Source: three-view drawing plus pictorial views. Frame: mm from the lowest corner of the part. Coordinates: 2 decimals unless noted, no trailing zeros. Order: outer loops, then holes, each group sorted by start corner. A loop starts at its lowest first (then second) coordinate and runs counter-clockwise, first axis right, second up. Notation, with made-up numbers: (81.5, -15) - (117.5, -15) arc R12 cw to (117.5, -1) - close; hole circle Ø4 at (-38, 64). An arc over 180 degrees is marked (long way). Use a Markdown table: item, result. Add a question column.
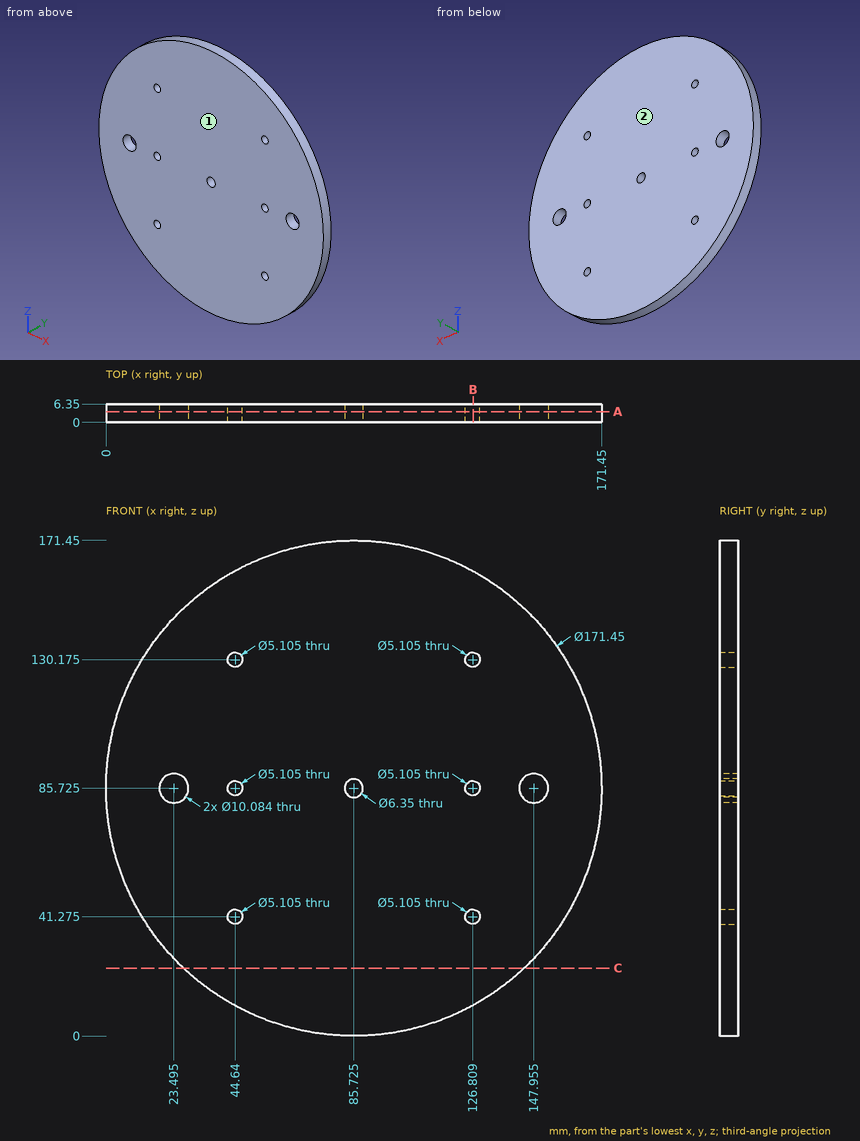
1) Section A-A (y = 3.75). Give the number of separate pieces and of enclosed holes in the cut face, then the cut area to 3 significant figures.
2) Section C-C (z = 23.5). Return loops of the section in (x, y), then the cut area to 3 significant figures.
3) Ray query, line 1 along X through (y, z) = (3, 43) (1 decimal); line 2 along X through (y, z) = (5, 130.5); line 3 along Z through (x, y) = (25, 5.75) (1 decimal). Return the intervals inside material, ascending.
4) Pin query (flat end, axial travel): pin 1 (1 mm diameter, centred on y = 4.5, z = 94.5, fed in from -X); pin 2 (3 mm diameter, centred on x = 107, y = 5.5, fed in from -Z); pin 3 (2 mm diameter, centred on x = 33.5, y = 2.5, fed in from +Z). Return the tip coordinate at first contact, or that it passes through.
5) Draft query along Y for the marked faces 1 and 2. Return one class per face: pulls with the +Y half, pulls with the -Y half, needs draft (parallel to the pull), parting line crosses it, or undercut.
6) Section B-B (x = 127). Return loops of the section in (y, z).
Values follow:
| question | item | result |
|---|---|---|
| 1 | separate pieces | 1 |
| 1 | enclosed holes | 9 |
| 1 | area | 22,800 mm² |
| 2 | outline | (26.76, 0) - (144.69, 0) - (144.69, 6.35) - (26.76, 6.35) - close |
| 2 | area | 749 mm² |
| 3 | line 1 | x = 11.4 to 42.8, 46.5 to 124.9, 128.7 to 160 |
| 3 | line 2 | x = 12.62 to 42.11, 47.17 to 124.28, 129.34 to 158.83 |
| 3 | line 3 | z = 25.2 to 80.9, 90.5 to 146.2 |
| 4 | pin 1 | stops at x = 0.4 |
| 4 | pin 2 | stops at z = 2.31 |
| 4 | pin 3 | stops at z = 154.46 |
| 5 | face 1 | pulls with the -Y half |
| 5 | face 2 | pulls with the +Y half |
| 6 | outline | (0, 10.59) - (6.35, 10.59) - (6.35, 38.73) - (0, 38.73) - close; (0, 43.82) - (6.35, 43.82) - (6.35, 83.18) - (0, 83.18) - close; (0, 88.27) - (6.35, 88.27) - (6.35, 127.63) - (0, 127.63) - close; (0, 132.72) - (6.35, 132.72) - (6.35, 160.86) - (0, 160.86) - close |
